from build123d import *


with BuildPart() as f1:
    # F0 (on Front) → F1 (revolve)
    with BuildSketch(Plane.XZ):
        with BuildLine():
            Line((-26.6725718975, -75.5722820759), (0, -75.5722820759))
            Line((0, -75.5722820759), (0, 15.8257279545))
            add(Edge.make_bspline(
                [(-11.0246650875, 68.8152387738), (-13.0319182183, 61.6892423346), (-17.1020054937, 47.2399299955), (-27.4894427467, 15.6142705276), (-8.8924216575, 15.7573246544), (0, 15.8257279545)],
                knots=[0, 0, 0, 0, 0.3367714548, 0.6828681405, 1, 1, 1, 1], degree=3))
            Line((-11.0246650875, 68.8152387738), (-17.7817139775, 68.8152387738))
            add(Edge.make_bspline(
                [(-4.9788798206, 6.9348705001), (-14.7560330129, 8.6892290012), (-35.3441774531, 12.3834522081), (-27.5698066923, 49.9831757822), (-20.8500701315, 62.9117928158), (-17.7817139775, 68.8152387738)],
                knots=[0, 0, 0, 0, 0.3294975078, 0.6938361452, 1, 1, 1, 1], degree=3))
            Line((-4.9788798206, 6.9348705001), (-4.9788798206, -71.6603025794))
            Line((-4.9788798206, -71.6603025794), (-26.6725718975, -71.6603025794))
            Line((-26.6725718975, -71.6603025794), (-26.6725718975, -75.5722820759))
        make_face()
    revolve(axis=Axis((0, 0, -1.244712621), (0, 0, -1)))


solid = f1.part
Work out the finished part from the listing and answer in its coordinate system (mm). A direction names the side the tool comes from. Give positions to 0.01 mm unless a question says otherwise; leave off trailing zeros. Loops run counter-clockwise (first coordinate to the right, second up) from the corner with the lowest first, then second, coordinate; pieces in that order, holes last. Notation, with made-up numbers: (77.5, 71) - (96.5, 71) arc R21 ccw to (96.5, 85) - close; hole circle Ø3 at (-30.75, 54). An arc over 180 degrees is marked (long way). Answer in a Markdown table with one row per item. Add a question column.
Q1. The part is cut by section B-B (z = -54.5). Determine the outline of the cut face in (x, y).
Q2. A tool of negligible diameter and unlimited length cuts with its end or side. For faces 4 (the cylindrical face through (1.08, -4.86, -32.91)), 5 (the cylindrical face through (-24.639, -10.216, -73.644)), from which of +Z, -Z, +X, -X, +Y, -Y can it reach the whole face along a straight path? Write none if from no direction.
Q3. Determine the mould class of faces 1 (the flat face through (-8, -8, 68.815)), 2 (the flat face through (6, 0, -71.66)), 3 (the flat face through (0, 0, -75.572)) for opening direction Z: released by +Z, released by -Z, zero draft, split by the parting line, or undercut.
Q4. Consider line 1 along Y through (x, z) = (-17, 36.5); line 2 along X through (y, z) = (-11, 45); line 3 along Z through (x, y) = (-2, 10). Determine where each line is inside the solid, lowest interval first.
Q5. Each of these flat-tipped pins is pushed along its axis until it touches: P1, Ø6, axis at x = 3, z = 51, coming from the +Y side; P2, Ø1.5, axis at y = 1.5, z = 20.5, coming from the -X side; P3, Ø2, axis at x = 1, z = -0.5, coming from the -Y side. Where does it stop, or does it pass through?
Q6. The part is cut by section A-A (y = -13). State how many separate pieces and enclosed holes the cut face has, and give its area (3 significant figures).
Solution:
| question | item | result |
|---|---|---|
| 1 | outline | circle Ø9.96 at (0, 0) |
| 2 | face 4 | none |
| 2 | face 5 | -Z |
| 3 | face 1 | released by +Z |
| 3 | face 2 | undercut |
| 3 | face 3 | released by -Z |
| 4 | line 1 | y = -24.43 to -11.47, 11.47 to 24.43 |
| 4 | line 2 | x = -25.49 to -14.25, 14.25 to 25.49 |
| 4 | line 3 | z = -75.57 to -71.66, 7.91 to 16.04 |
| 5 | P1 | stops at y = 26.72 |
| 5 | P2 | stops at x = -29.96 |
| 5 | P3 | stops at y = -4.98 |
| 6 | separate pieces | 2 |
| 6 | enclosed holes | 1 |
| 6 | area | 1,740 mm² |
